```python
from build123d import *

# Parameters (mm, degrees)
F0_R     = 31.75
F2_DEPTH = 10.16
F3_D     = 20.32
F4_R     = 5.08
F5_R     = 5.07999


# Not quite as in the source:
# - a fillet or chamfer is up to 0.001 mm smaller than in the source, because OpenCascade refuses the exact size


with BuildPart() as f2:
    # F0 (on Right) → F2 (new body)
    with BuildSketch(Plane.YZ):
        Circle(F0_R)
    extrude(amount=F2_DEPTH)

    # F3 (through all)
    with Locations(Plane(origin=(0, 0, 0), x_dir=(0, 1, 0), z_dir=(-1, 0, 0))):
        with Locations((0, 0)):
            Hole(F3_D / 2)

    # F4
    f4_edges = [f2.edges().sort_by_distance(p)[0] for p in [
        (0, -31.75, 0),
    ]]
    fillet(f4_edges, radius=F4_R)

    # F5 (radius 5.08 in the source; OpenCascade refuses exactly that, so slightly less here)
    f5_edges = [f2.edges().sort_by_distance(p)[0] for p in [
        (10.16, -31.75, 0),
    ]]
    fillet(f5_edges, radius=F5_R)


solid = f2.part
```
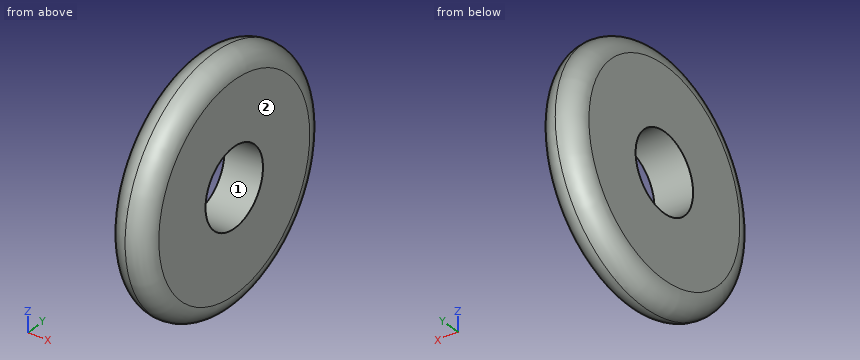
Could you check a few things on this model? Use its own coordinates, in mm. Face numbers are marked on the shaded views. Round coordinates to 2 decimals unless told otherwise and drop trailing zeros. Loops run counter-clockwise (first coordinate to the right, second up) from the corner with the lowest first, then second, coordinate; pieces in that order, holes last. Notation, with made-up numbers: (53, 58.5) -> (107, 58.5) arc R19 cw to (107, 87.5) -> close; hole circle Ø8 at (-35.5, 74). An arc over 180 degrees is marked (long way). Put each result on its own line as item: value.
Q1. Thinking about a two-plate mould opening in Z: for the marked faces 1 and 2, which applies, pulls with the +Z half, pulls with the -Z half, needs draft (parallel to the pull), parting line crosses it, or undercut?
Checks:
face 1: undercut
face 2: needs draft
Q2. I want a section at C-C on x = 7.5. Write out the boundary of the cut face in (y, z), and give its area (3 significant figures).
Checks:
outline: circle Ø62.27 at (0, 0); hole circle Ø20.32 at (0, 0)
area: 2,720 mm2
Q3. Please list where these lines run through material, in increasing order: line 1 (Y direction, x = 2, z = -5); line 2 (Z direction, x = 7.25, y = 0); line 3 (X direction, y = -14.5, z = -27). Write a range as from..to.
Checks:
line 1: -30.3..-8.84, 8.84..30.3
line 2: -31.26..-10.16, 10.16..31.26
line 3: 1.92..8.24
Q4. For pin 1 Ø1 at (x, y) = (3.5, -2) entering from +Z; pin 2 Ø3 at (x, z) = (1.5, -9.5) entering from +Y; pin 3 Ø1 at (x, z) = (4.5, 5) entering from +Y, each with a flat end and sliding along its axis, tell me the tip position at first contact or that it passes through.
Checks:
pin 1: z = 31.57
pin 2: y = 29.96
pin 3: y = 31.41
Q5. I want a section at D-D on x = 3. Write out the boundary of the cut face in (y, z), and give its area (3 significant figures).
Checks:
outline: circle Ø62.61 at (0, 0); hole circle Ø20.32 at (0, 0)
area: 2,750 mm2
